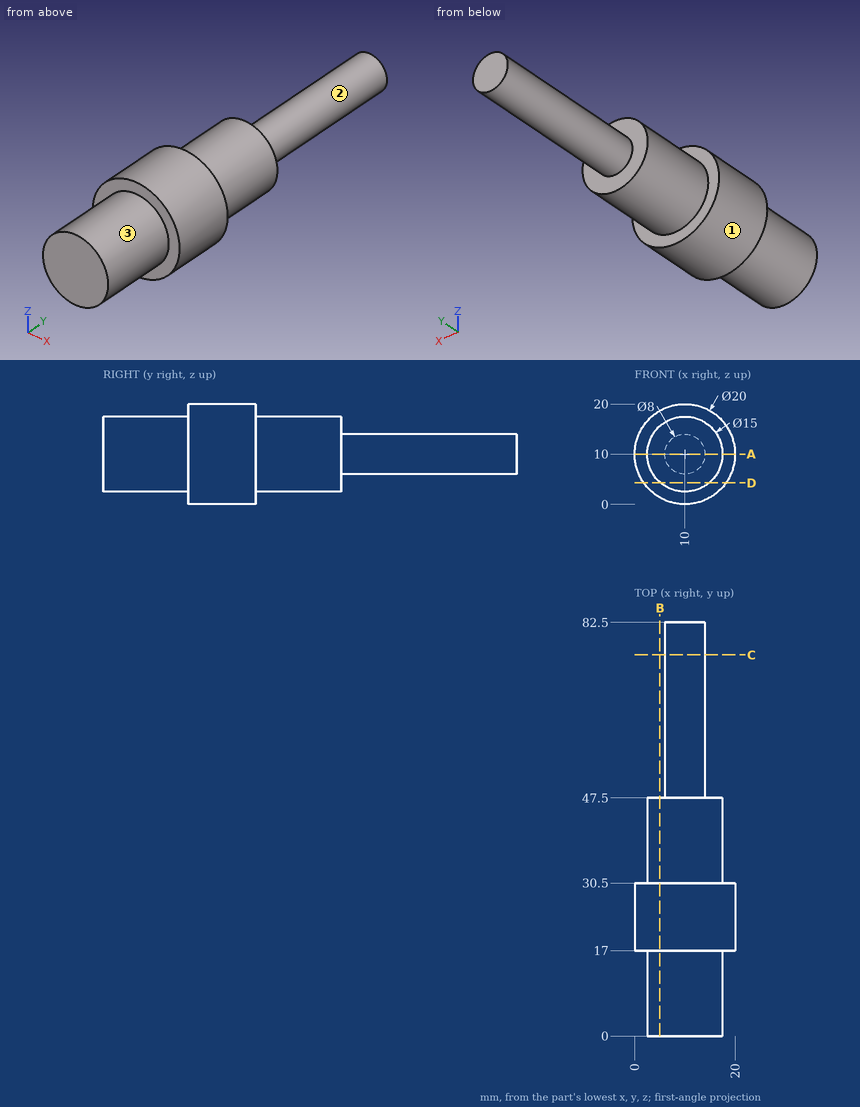
The figure shows three views and two pictorial views of one solid part (mm, origin at its lowest corner). Answer the questions. A direction names the side the tool comes from. Coordinates: 2 decimals unless noted, no trailing zeros. Loops run counter-clockwise (first coordinate to the right, second up) from the corner with the lowest first, then second, coordinate; pieces in that order, holes last. Notation, with made-up numbers: (-11, 27.25) -> (12, 27.25) arc R13 cw to (12, 37.25) -> close; hole circle Ø10 at (32, -30). An arc over 180 degrees is marked (long way). Return JSON: item names as keys, results as strings. Group by question number.
(1) Find the intervals of material crossed by probe 1 along Y at (x, z) = (8.5, 18); probe 2 along Y at (x, z) = (4.5, 12.75); probe 3 along Z at (x, y) = (4.5, 28.5), in increasing order. Write a range as from..to.
(2) A cutting plane is placed at A-A on z = 10. Write down the section's boundary in (x, y), and give its area (3 significant figures).
(3) A cutting plane is placed at B-B on x = 5. Write down the section's boundary in (y, z), and give its area (3 significant figures).
(4) A cutting plane is placed at C-C on y = 76. Write down the section's boundary in (x, z).
(5) Given pin 1 Ø2 at (y, z) = (38, 10) entering from -X; pin 2 Ø5 at (y, z) = (46.5, 7.5) entering from +X; pin 3 Ø8 at (y, z) = (14.5, 3) entering from -X, each flat-ended and moving along its own axis, determine where each tip first touches the part or whether it passes through.
(6) A cutting plane is placed at D-D on z = 4.25. Write down the section's boundary in (x, y).
(7) Which of the six approach directions +Z, -Z, +X, -X, +Y, -Y give full straight-line access (tool end or side, diameter ignored) to the marked faces 1, 2 and 3?
The answers:
{
 "1": {"probe 1": "y = 17..30.5", "probe 2": "y = 0..47.5", "probe 3": "z = 1.65..18.35"},
 "2": {"outline": "(0, 17) -> (2.5, 17) -> (2.5, 0) -> (17.5, 0) -> (17.5, 17) -> (20, 17) -> (20, 30.5) -> (17.5, 30.5) -> (17.5, 47.5) -> (14, 47.5) -> (14, 82.5) -> (6, 82.5) -> (6, 47.5) -> (2.5, 47.5) -> (2.5, 30.5) -> (0, 30.5) -> close", "area": "1,060 mm^2"},
 "3": {"outline": "(0, 4.41) -> (17, 4.41) -> (17, 1.34) -> (30.5, 1.34) -> (30.5, 4.41) -> (47.5, 4.41) -> (47.5, 15.59) -> (30.5, 15.59) -> (30.5, 18.66) -> (17, 18.66) -> (17, 15.59) -> (0, 15.59) -> close", "area": "614 mm^2"},
 "4": {"outline": "circle Ø8 at (10, 10)"},
 "5": {"pin 1": "stops at x = 2.5", "pin 2": "stops at x = 17.5", "pin 3": "stops at x = 0.78"},
 "6": {"outline": "(1.82, 17) -> (5.18, 17) -> (5.18, 0) -> (14.82, 0) -> (14.82, 17) -> (18.18, 17) -> (18.18, 30.5) -> (14.82, 30.5) -> (14.82, 47.5) -> (5.18, 47.5) -> (5.18, 30.5) -> (1.82, 30.5) -> close"},
 "7": {"face 1": "+Y, -Y", "face 2": "+Y", "face 3": "-Y"}
}
